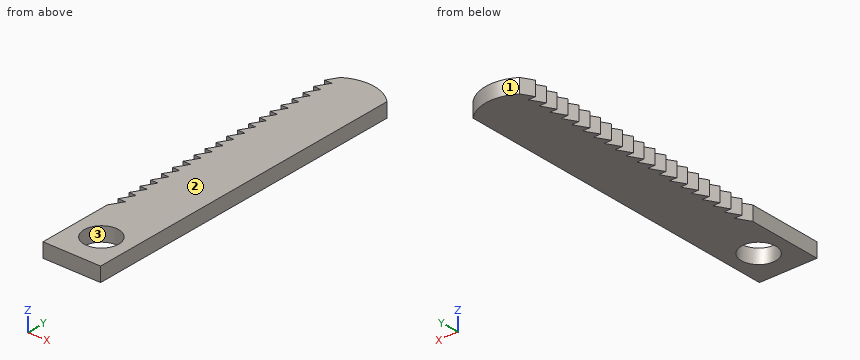
from build123d import *

# Parameters (mm, degrees)
ESQUISSE1_R                = 3
BASE_EXTRUSION_DEPTH       = 2.5
ENL_V_MAT_EXTRU_1_DEPTH    = 102.356317555
R_P_TITION_LIN_AIRE1_COUNT = 22
R_P_TITION_LIN_AIRE1_PITCH = 2.2


with BuildPart() as part:
    # Esquisse1 → Base-Extrusion (new body)
    with BuildSketch(Plane.XY):
        with BuildLine():
            Line((-5, 99.101020514), (-5, 41.101020514))
            Line((-5, 41.101020514), (5, 41.101020514))
            Line((5, 41.101020514), (5, 99.101020514))
            ThreePointArc((5, 99.101020514), (0, 101.202041029), (-5, 99.101020514))
        make_face()
        with Locations((0, 47.101020514)):
            Circle(ESQUISSE1_R, mode=Mode.SUBTRACT)
    extrude(amount=BASE_EXTRUSION_DEPTH)

    # Esquisse2 → Enlèv. mat.-Extru.1 (cut, through all)
    with BuildSketch(Plane.XY.offset(2.5)):
        Polygon((-5, 56.301020514), (-5, 54.101020514), (-3.729829408, 56.301020514), align=None)
    enl_v_mat_extru_1 = extrude(amount=-ENL_V_MAT_EXTRU_1_DEPTH, mode=Mode.SUBTRACT)

    # Répétition linéaire1: Enlèv. mat.-Extru.1 ×22
    with Locations(*[(0, i * R_P_TITION_LIN_AIRE1_PITCH, 0) for i in range(1, R_P_TITION_LIN_AIRE1_COUNT)]):
        add(enl_v_mat_extru_1, mode=Mode.SUBTRACT)


solid = part.part
Part model, mm, in its own coordinate system. Face numbers are marked on the shaded views. Give positions to 0.01 mm unless a question says otherwise; leave off trailing zeros. Loops run counter-clockwise (first coordinate to the right, second up) from the corner with the lowest first, then second, coordinate; pieces in that order, holes last. Notation, with made-up numbers: M 58.5,89.25 L 99.5,89.25 A12 cw 99.5,98.25 Z; hole C 53.25,1.5 d5. An arc over 180 degrees is marked long. Put each result on its own line as item: value. Start each with the question number.
1) Saw through at A-A (x = 0). List the corners of the cut face in (y, z), then the cut area to 3 significant figures.
2) Saw through at C-C (x = 4). List the corners of the cut face in (y, z), then the cut area to 3 significant figures.
3) Saw through at B-B (y = 61.5). List the corners of the cut face in (x, z).
4) Probe probe 1 along Y at (x, z) = (0, 1.05); probe 2 along Y at (x, z) = (0.75, 2.4); probe 3 along X at (y, z) = (67, 2.05). List the from-to ranges inside material, lowest first.
5) Pull direction Y, two halves, no side cores. Call the marked faces 1, 2 and 3: +Y half, -Y half, draft (parallel to the pull), parting line (faces both ways), or undercut.
Numbers:
1. outline: M 41.1,0 L 44.1,0 L 44.1,2.5 L 41.1,2.5 Z; M 50.1,0 L 101.2,0 L 101.2,2.5 L 50.1,2.5 Z
1. area: 135 mm^2
2. outline: M 41.1,0 L 99.95,0 L 99.95,2.5 L 41.1,2.5 Z
2. area: 147 mm^2
3. outline: M -4.54,0 L 5,0 L 5,2.5 L -4.54,2.5 Z
4. probe 1: 41.1 to 44.1, 50.1 to 101.2
4. probe 2: 41.1 to 44.2, 50.01 to 101.16
4. probe 3: -3.9 to 5
5. face 1: +Y half
5. face 2: draft
5. face 3: undercut
